Design review of the part shown in the three views and the two pictorial views. Dimensions are in mm from the part's minimum x, y and z. A direction names the side the tool comes from. Coordinates: 2 decimals unless noted, no trailing zeros. Loops run counter-clockwise (first coordinate to the right, second up) from the corner with the lowest first, then second, coordinate; pieces in that order, holes last. Notation, with made-up numbers: M 9,-33 L 44,-33 A35 cw 44,5 Z; hole C 43.25,40.25 d8. An arc over 180 degrees is marked long. Put each result on its own line as item: value. Start each with the question number.
(1) For probe 1 along X at (y, z) = (17.25, 7.5); probe 2 along Z at (x, y) = (49, 4), list the stretches that pass through material, from the lowest coordinate up. Write a range as [from, to].
(2) Take a section at B-B, the plane y = 19. Give the boundary of the cut face in (x, z).
(3) Take a section at C-C, the plane x = 47. Give the boundary of the cut face in (y, z).
(4) Take a section at A-A, the plane z = 10.5. Give the boundary of the cut face in (x, y).
(5) For the marked faces 4 and 5, list the 3-axis set-ups (+Z, -Z, +X, -X, +Y, -Y) from which the entire face can be reached by the end or side of a thin tool; tool diameter is ignored.
(6) The part is to be moulded in two halves that separate along X. For the marked faces 1, 2 and 3, say which applies: +X half, -X half, draft (parallel to the pull), parting line (faces both ways), or undercut.
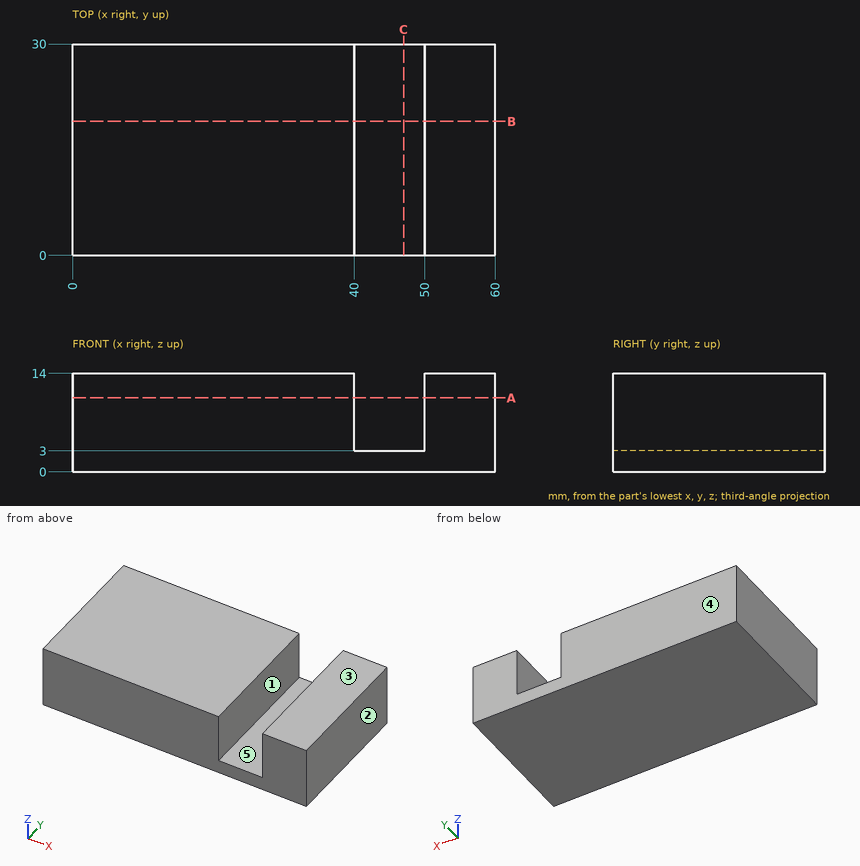
Computed values:
1. probe 1: x = [0, 40], [50, 60]
1. probe 2: z = [0, 3]
2. outline: M 0,0 L 60,0 L 60,14 L 50,14 L 50,3 L 40,3 L 40,14 L 0,14 Z
3. outline: M 0,0 L 30,0 L 30,3 L 0,3 Z
4. outline: M 0,0 L 40,0 L 40,30 L 0,30 Z; M 50,0 L 60,0 L 60,30 L 50,30 Z
5. face 4: +Z, -Z, +X, -X, +Y
5. face 5: +Z, +Y, -Y
6. face 1: undercut
6. face 2: +X half
6. face 3: draft
